```python
from build123d import *

# Parameters (mm, degrees)
F4_R = 0.5
F5_R = 0.5
F6_R = 0.5


# Not quite as in the source:
# - a feature of the source that left no trace in its solid (it failed there, or was rolled back) is left out


with BuildPart() as f1:
    # F0 (on Front) → F1 (revolve)
    with BuildSketch(Plane.XZ):
        Polygon((-2.1, -3), (-8.9066560708, 0), (-11.6, 0), (-11.6, -5), (-5.6, -5), (-5.6, -3.5), (-2.1, -3.5), align=None)
        Polygon((-11.6, 0), (-8.9066560708, 0), (-12.1, 1.4074505437), (-13.6, 1.4074505437), (-13.6, 2.9074505437), (-17.5, 2.9074505437), (-17.5, 2), (-14.1, 2), (-14.1, 0), align=None)
    revolve(axis=Axis((0, 0, -7.5), (0, 0, -1)))

    # F4
    f4_edges = [f1.edges().sort_by_distance(p)[0] for p in [
        (13.6, 0, 1.407451),
    ]]
    fillet(f4_edges, radius=F4_R)

    # F5
    f5_edges = [f1.edges().sort_by_distance(p)[0] for p in [
        (12.1, 0, 1.407451),
    ]]
    fillet(f5_edges, radius=F5_R)

    # F6
    f6_edges = [f1.edges().sort_by_distance(p)[0] for p in [
        (13.6, 0, 2.907451),
    ]]
    fillet(f6_edges, radius=F6_R)


solid = f1.part
```
Source: CAD feature listing. Evaluate the final solid. Frame: model axes, mm. A direction names the side the tool comes from. Give positions to 0.01 mm unless a question says otherwise; leave off trailing zeros. Loops run counter-clockwise (first coordinate to the right, second up) from the corner with the lowest first, then second, coordinate; pieces in that order, holes last. Notation, with made-up numbers: (54, -17) - (102, -17) arc R6 cw to (102, -8) - close; hole circle Ø2 at (7.5, 67.5). An arc over 180 degrees is marked (long way). Use CSV: the item, a comma, the result in double quotes.
1) Mould query, pull axis Y, two halves, no side actions, for faces 1 (the cylindrical face through (-6.506, -12.509, 0.986)), 2 (the cylindrical face through (2.948, -13.277, 2.161)), 3 (the flat face through (12, 8, 2)). Classes: +Y half, -Y half, draft (parallel to the pull), parting line (faces both ways), or undercut.
Worked out:
face 1,"parting line"
face 2,"undercut"
face 3,"draft"
2) Pin query (flat end, axial travel): P1, Ø1.5, axis at x = 1, z = -2, coming from the -Y side; P2, Ø9, axis at x = 0, y = 0, coming from the -Z side; P3, Ø6, axis at x = 8, y = 7.5, coming from the +Z side. Return the tip coordinate at first contact, or that it passes through.
Worked out:
P1,"stops at y = -11.6"
P2,"stops at z = -3.5"
P3,"stops at z = 2.89"
3) Cut plane A-A (z = -1.25). Output: boundary loops of the cut face in (x, y).
Worked out:
outline,"circle Ø23.2 at (0, 0); hole circle Ø12.14 at (0, 0)"
4) Line query: line 1 (Y direction, x = 0, z = -4.3); line 2 (Y direction, x = 0, z = -3.3); line 3 (Z direction, x = 3, y = 15.5). Output: solid intervals per line, ascending.
Worked out:
line 1,"y = -11.6 to -5.6, 5.6 to 11.6"
line 2,"y = -11.6 to -2.1, 2.1 to 11.6"
line 3,"z = 2 to 2.91"
5) Set-up query: faces 4 (the cylindrical face through (5.595, 0.246, -4.24)), 5 (the flat face through (-12, 8, 2.907)), 6 (the flat face through (-6, 11, 1.407)). Return all of +Z, -Z, +X, -X, +Y, -Y with unobstructed straight access to the full face (end or side cutting, diameter ignored); none if empty.
Worked out:
face 4,"-Z"
face 5,"+Z, +X, -X, +Y, -Y"
face 6,"+Z"
